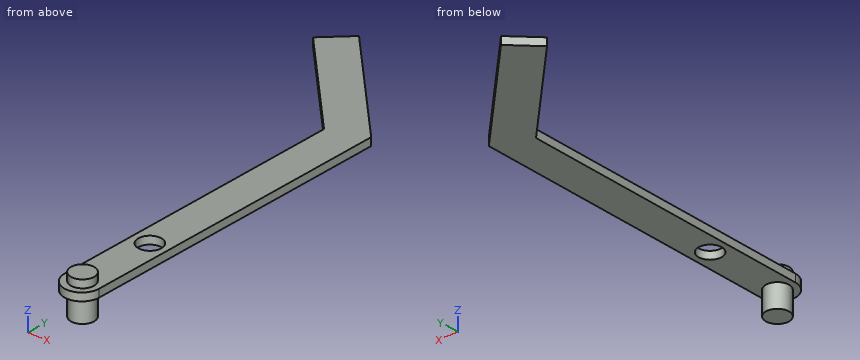
```python
from build123d import *

# Parameters (mm, degrees)
SKETCH_1_R           = 3
EXTRUDE_1_DEPTH      = 2
SKETCH_2_R           = 3
EXTRUDE_2_DEPTH      = 2
EXTRUDE_2_DEPTH_BACK = 8
EXTRUDE_4_DEPTH      = 2
SCALE_1_SCALE        = 3.5


with BuildPart() as part:
    # 草图1 → 凸台-拉伸1 (new body)
    with BuildSketch(Plane.XY):
        with BuildLine():
            Line((-4.5, -20), (-4.5, 20))
            ThreePointArc((-4.5, 20), (0, 24.5), (4.5, 20))
            Line((4.5, 20), (4.5, -20))
            ThreePointArc((4.5, -20), (0, -24.5), (-4.5, -20))
        make_face()
        Circle(SKETCH_1_R, mode=Mode.SUBTRACT)
    extrude(amount=EXTRUDE_1_DEPTH)

    # 草图2 → 凸台-拉伸2 (add, two sides)
    with BuildSketch(Plane.XY.offset(2)) as extrude_2_sk:
        with Locations((0, -19.804668681)):
            Circle(SKETCH_2_R)
    extrude(amount=EXTRUDE_2_DEPTH)
    extrude(extrude_2_sk.sketch, amount=-EXTRUDE_2_DEPTH_BACK)

    # 草图3 → 凸台-拉伸4 (add)
    with BuildSketch(Plane.XY.offset(2)):
        Polygon((-4.5, 20), (-4.5, 56.272077939), (-30.148232278, 81.920310217), (-23.784271247, 88.284271247), (4.5, 60), (4.5, 20), align=None)
    extrude(amount=-EXTRUDE_4_DEPTH)


with BuildPart() as part_1:
    # 缩放比例1: scaled about (-3.938760867, 30.155336672, 0.75690128)
    add(part.part.scale(SCALE_1_SCALE).moved(Location((9.846902167, -75.38834168, -1.8922532))))


solid = part_1.part
```
Here's how the part is built. I have some questions about the finished solid (model axes, mm). Coordinates: 2 decimals unless noted, no trailing zeros. Order: outer loops, then holes, each group sorted by start corner. A loop starts at its lowest first (then second) coordinate and runs counter-clockwise, first axis right, second up.
Item 1: If we section it at C-C, the plane x = -65: List the corners of the cut face in (y, z) for me, then the cut area to 3 significant figures.
Response values:
outline: (180.66, -1.89) - (225.21, -1.89) - (225.21, 5.11) - (180.66, 5.11) - close
area: 312 mm2
Item 2: If we section it at A-A, the plane y = -101: List the corners of the cut face in (x, z) for me, then the cut area to 4 significant figures.
Response values:
outline: (-5.9, -1.89) - (25.6, -1.89) - (25.6, 5.11) - (-5.9, 5.11) - close
area: 220.5 mm2
Item 3: I need wall thicknesses on probe 1 along X at (y, z) = (5, 0); probe 2 along Z at (x, y) = (16, 6.5); probe 3 along Y at (x, z) = (18.5, 4). Which ranges of each line are inside material? Lowest first, please.
Response values:
probe 1: x = -5.9 to 25.6
probe 2: z = -1.89 to 5.11
probe 3: y = -158.55 to -81.34, -69.44 to 141.71
Item 4: I'm going to push flat-ended pins straight in: pin 1 Ø4 at (x, y) = (7, 27.5) entering from +Z; pin 2 Ø1 at (y, z) = (187.5, 2) entering from -X; pin 3 Ø5 at (x, z) = (-1.5, 4.5) entering from -Y. Where does each tip first touch, or does it pass through?
Response values:
pin 1: stops at z = 5.11
pin 2: stops at x = -72.34
pin 3: stops at y = -158.42
Item 5: If we section it at B-B, the plane z = 8.5: List the corners of the cut face in (x, y) for me, then the cut area to 3 significant figures.
Response values:
outline: circle Ø21 at (9.85, -144.7)
area: 346 mm2
